from build123d import *

# Parameters (mm, degrees)
BOSS_EXTRUDE2_DEPTH     = 69.5
BOSS_EXTRUDE3_DEPTH     = 69.5
CUT_EXTRUDE1_DEPTH      = 77.399445549
CUT_EXTRUDE1_DEPTH_BACK = 77.399445549
SKETCH7_R               = 2
CUT_EXTRUDE2_DEPTH      = 78.109924218
CUT_EXTRUDE2_DEPTH_BACK = 78.109924218
SKETCH8_R               = 1.7
FILLET1_R               = 0.2
BOSS_EXTRUDE4_DEPTH     = 2.5


with BuildPart() as part:
    # Sketch4 → Boss-Extrude2 (new body)
    with BuildSketch(Plane.XY):
        Polygon((-10.152602112, 10.223468411), (-10.152602112, -5.476531589), (-4.682602112, -5.476531589), (-4.682602112, -2.436531589), (-5.282780111, -2.436531589), (-6.782780111, -3.556531589), (-7.782602112, -3.556531589), (-7.782602112, 8.303468411), (-6.782780111, 8.303468411), (-5.282780111, 7.183468411), (-4.682602112, 7.183468411), (-4.682602112, 10.223468411), align=None)
    extrude(amount=BOSS_EXTRUDE2_DEPTH)

    # Sketch6 → Boss-Extrude3 (add)
    with BuildSketch(Plane.XY.offset(69.5)):
        with BuildLine():
            Line((-18.82375255, 27.373468411), (-23.82375255, 27.373468411))
            Line((-23.82375255, 27.373468411), (-23.82375255, 15.03032266))
            ThreePointArc((-23.82375255, 15.03032266), (-23.51927068, 13.499588931), (-22.652179675, 12.201895535))
            Line((-22.652179675, 12.201895535), (-20.82375255, 10.373468411))
            Line((-20.82375255, 10.373468411), (-20.82375255, -5.626531589))
            Line((-20.82375255, -5.626531589), (-22.652179675, -7.454958714))
            ThreePointArc((-22.652179675, -7.454958714), (-23.51927068, -8.752652109), (-23.82375255, -10.283385839))
            Line((-23.82375255, -10.283385839), (-23.82375255, -22.626531589))
            Line((-23.82375255, -22.626531589), (-18.82375255, -22.626531589))
            Line((-18.82375255, -22.626531589), (-18.82375255, -11.458931103))
            ThreePointArc((-18.82375255, -11.458931103), (-18.088209901, -9.14736925), (-16.152093449, -7.685933561))
            Line((-16.152093449, -7.685933561), (-10.152602112, -5.476531589))
            Line((-10.152602112, -5.476531589), (-10.152602112, 10.223468411))
            Line((-10.152602112, 10.223468411), (-16.820008224, 12.668019889))
            ThreePointArc((-16.820008224, 12.668019889), (-18.272095564, 13.764096656), (-18.82375255, 15.497768046))
            Line((-18.82375255, 15.497768046), (-18.82375255, 27.373468411))
        make_face()
    extrude(amount=-BOSS_EXTRUDE3_DEPTH)

    # Sketch7 → Cut-Extrude1 (cut, two sides: drawn at the far end of the back side and taken through both)
    with BuildSketch(Plane(origin=(-7.782602112, 0, 0), x_dir=(0, 0, -1), z_dir=(1, 0, 0)).offset(-CUT_EXTRUDE1_DEPTH_BACK)):
        with Locations(Location((-34.5, 2.373468411, 0), (0, 0, 180))):
            Circle(SKETCH7_R)
        with Locations(Location((-14.5, 2.373468411, 0), (0, 0, 180))):
            Circle(SKETCH7_R)
    extrude(amount=CUT_EXTRUDE1_DEPTH + CUT_EXTRUDE1_DEPTH_BACK, mode=Mode.SUBTRACT)

    # Sketch8 → Cut-Extrude2 (cut, two sides: drawn at the far end of the back side and taken through both)
    with BuildSketch(Plane.ZY.offset(23.82375255).offset(-CUT_EXTRUDE2_DEPTH_BACK)):
        with Locations(Location((57.5, 19.373468411, 0), (0, 0, 270))):
            Circle(SKETCH8_R)
        with Locations(Location((57.5, -14.626531589, 0), (0, 0, 270))):
            Circle(SKETCH8_R)
        with BuildLine():
            Line((15.4, 21.073468411), (8.6, 21.073468411))
            ThreePointArc((8.6, 21.073468411), (6.9, 19.373468411), (8.6, 17.673468411))
            Line((8.6, 17.673468411), (15.4, 17.673468411))
            ThreePointArc((15.4, 17.673468411), (17.1, 19.373468411), (15.4, 21.073468411))
        make_face()
        with BuildLine():
            Line((8.6, -12.926531589), (15.4, -12.926531589))
            ThreePointArc((15.4, -12.926531589), (17.1, -14.626531589), (15.4, -16.326531589))
            Line((15.4, -16.326531589), (8.6, -16.326531589))
            ThreePointArc((8.6, -16.326531589), (6.9, -14.626531589), (8.6, -12.926531589))
        make_face()
    extrude(amount=CUT_EXTRUDE2_DEPTH + CUT_EXTRUDE2_DEPTH_BACK, mode=Mode.SUBTRACT)

    # Fillet1
    fillet1_edges = [part.edges().sort_by_distance(p)[0] for p in [
        (-4.682602112, 7.183468411, 34.75),
        (-5.282780111, 7.183468411, 34.75),
        (-5.282780111, -2.436531589, 34.75),
        (-4.682602112, -2.436531589, 34.75),
    ]]
    fillet(fillet1_edges, radius=FILLET1_R)

    # Sketch9 → Boss-Extrude4 (add)
    with BuildSketch(Plane.XY.offset(69.5)):
        Polygon((-7.782602112, 8.303468411), (-7.782602112, -3.556531589), (-6.782780111, -3.556531589), (-5.336008623, -2.476275545), (-5.336008623, 7.223212366), (-6.782780111, 8.303468411), align=None)
    extrude(amount=-BOSS_EXTRUDE4_DEPTH)


solid = part.part
Verification items for the finished model (mm, model axes). A direction names the side the tool comes from. Round coordinates to 2 decimals unless told otherwise and drop trailing zeros. Loops run counter-clockwise (first coordinate to the right, second up) from the corner with the lowest first, then second, coordinate; pieces in that order, holes last. Notation, with made-up numbers: (41, 57) - (57, 57) arc R15 ccw to (57, 75) - close; hole circle Ø4 at (88.25, 24). An arc over 180 degrees is marked (long way). Write item = value, one per line.
Q1. Sectioned sample at C-C on y = 19.5. Record the boundary of the cut face in (x, z).
Here are the results:
outline = (-23.82, 0) - (-18.82, 0) - (-18.82, 6.9) - (-23.82, 6.9) - close; (-23.82, 17.1) - (-18.82, 17.1) - (-18.82, 55.8) - (-23.82, 55.8) - close; (-23.82, 59.2) - (-18.82, 59.2) - (-18.82, 69.5) - (-23.82, 69.5) - close
Q2. Material ranges on L1, parallel to Y at x = -20.1, z = 57.5; L2, parallel to Z at x = -21.25, y = -15; L3, parallel to X at y = -0.5, z = 34, recorded low to high.
Here are the results:
L1 = -22.63 to -16.33, -12.93 to 17.67, 21.07 to 27.37
L2 = 0 to 6.94, 17.06 to 55.84, 59.16 to 69.5
L3 = -20.82 to -7.78
Q3. Sectioned sample at B-B on x = -13.5. Record the boundary of the cut face in (y, z).
Here are the results:
outline = (-6.71, 0) - (11.45, 0) - (11.45, 69.5) - (-6.71, 69.5) - close; hole circle Ø4 at (2.37, 14.5); hole circle Ø4 at (2.37, 34.5)
Q4. Mould release check, pull along Z, two halves, no side actions. Record for faces 1 (the flat face through (-21.7, -6.5, 35.2)), 2 (the flat face through (-17, 3, 69.5)), 3 (the cylindrical face through (-14.39, 1.02, 13.03)): +Z half, -Z half, draft (parallel to the pull), parting line (faces both ways), or undercut.
Here are the results:
face_1 = draft
face_2 = +Z half
face_3 = undercut
Q5. Tool access check on faces 4 (the flat face through (-5.336, 2, 68)), 5 (the cylindrical face through (-23.528, 13.52, 35.236)), 6 (the flat face through (-21, 17.673, 12)). Record the directions out of +Z, -Z, +X, -X, +Y, -Y that give a thin tool (end or side, any length) a straight path to the whole face; none if there is none.
Here are the results:
face_4 = +Z, -Z, +X
face_5 = +Z, -Z, -X
face_6 = +X, -X
Q6. Sectioned sample at D-D on z = 14.5. State how many separate pieces and enclosed holes the cut face has, plus the area to 3 significant figures.
Here are the results:
separate_pieces = 4
enclosed_holes = 0
area = 324 mm^2
Q7. Depth check by flat-ended pin: pin 1 (0.8 mm diameter, centred on x = -7.5, z = 24.5, fed in from +Y); pin 2 (2.5 mm diameter, centred on y = 2.37, z = 34.5, fed in from +X); pin 3 (8 mm diameter, centred on x = -8.5, z = 45, fed in from -Y); pin 4 (4.5 mm diameter, centred on y = 2.37, z = 14.5, fed in from -X). Enter the tip coordinate at first touch or a pass-through.
Here are the results:
pin_1 = 10.22
pin_2 = through
pin_3 = -6.34
pin_4 = -20.82
